from build123d import *

# Parameters (mm, degrees)
F0_W     = 28.575
F0_H     = 171.45
F0_R     = 1.5875
F1_DEPTH = 1.5875


with BuildPart() as f1:
    # F0 (on Front) → F1 (new body, symmetric)
    with BuildSketch(Plane.XZ):
        Rectangle(F0_W, F0_H)
        with Locations((-7.9375, -63.5)):
            Circle(F0_R, mode=Mode.SUBTRACT)
        with Locations((7.9375, -63.5)):
            Circle(F0_R, mode=Mode.SUBTRACT)
    extrude(amount=F1_DEPTH, both=True)


solid = f1.part
Work out the finished part from the listing and answer in its coordinate system (mm). Give positions to 0.01 mm unless a question says otherwise; leave off trailing zeros. Loops run counter-clockwise (first coordinate to the right, second up) from the corner with the lowest first, then second, coordinate; pieces in that order, holes last. Notation, with made-up numbers: (47, 87.25) - (59, 87.25) arc R15 ccw to (59, 104.25) - close; hole circle Ø4 at (-6, 6.5). An arc over 180 degrees is marked (long way). Answer in a Markdown table with one row per item. Add a question column.
Q1. Each of these flat-tipped pins is pushed along its axis until it touches: P1, Ø3.5, axis at x = 7.94, z = -63.5, coming from the -Y side; P2, Ø2.5, axis at x = -7.94, z = -63.5, coming from the +Y side. Where does it stop, or does it pass through?
Q2. Consider line 1 along Z through (x, y) = (8.75, -1.1) (3 decimals); line 2 along Z through (x, y) = (7.5, 1.05) (3 decimals). Determine where each line is inside the solid, lowest interval first.
Q3. The part is cut by section A-A (z = -63.5). State how many separate pieces and enclosed holes the cut face has, and give its area (3 significant figures).
Q4. Determine the mould class of faces 1 (the flat face through (14.288, 0, -1)), 2 (the flat face through (0, 0, -85.725)), 3 (the cylindrical face through (-8.144, 0.022, -61.926)) for opening direction X: released by +X, released by -X, zero draft, split by the parting line, or undercut.
Q5. The part is cut by section B-B (x = -7.75). Determine the outline of the cut face in (y, z) (1 decimal), and give its area (3 significant figures).
Solution:
| question | item | result |
|---|---|---|
| 1 | P1 | stops at y = -1.59 |
| 1 | P2 | passes through |
| 2 | line 1 | z = -85.725 to -64.864, -62.136 to 85.725 |
| 2 | line 2 | z = -85.725 to -65.026, -61.974 to 85.725 |
| 3 | separate pieces | 3 |
| 3 | enclosed holes | 0 |
| 3 | area | 70.6 mm² |
| 4 | face 1 | released by +X |
| 4 | face 2 | zero draft |
| 4 | face 3 | undercut |
| 5 | outline | (-1.6, -85.7) - (1.6, -85.7) - (1.6, -65.1) - (-1.6, -65.1) - close; (-1.6, -61.9) - (1.6, -61.9) - (1.6, 85.7) - (-1.6, 85.7) - close |
| 5 | area | 534 mm² |
